Design review of the part built by this model. Coordinates are the model's own, in mm. Face numbers are marked on the shaded views. A direction names the side the tool comes from. Coordinates: 2 decimals unless noted, no trailing zeros. Write each loop counter-clockwise with the first axis right and the second up, starting at its lowest first coordinate (ties: lowest second). Pieces come first, ordered by that corner, then holes. Notation, with made-up numbers: (-5, 56) - (24, 56) arc R18 ccw to (24, 76) - close; hole circle Ø9 at (73.25, 37). An arc over 180 degrees is marked (long way). Use a Markdown table: item, result.
from build123d import *

# Parameters (mm, degrees)
F3_DEPTH = 55.88
F4_COUNT = 15


with BuildPart() as f1:
    # F0 (on Front) → F1 (revolve)
    with BuildSketch(Plane.XZ):
        Polygon((-43.6586365104, 67.430395633), (-43.6586365104, 44.1211201251), (-7.5847627595, 44.1211201251), (-7.5847627595, 11.192150414), (-31.8190082908, 11.192150414), (-31.8190082908, -3.6073876545), (-21.0893414915, -3.6073876545), (-21.0893414915, -7.1222772822), (-15.1695264503, -7.1222772822), (-15.1695264503, -3.6073876545), (-8.6947288364, -3.6073876545), (-8.6947288364, -17.8519431502), (8.1397471949, -17.8519431502), (8.1397471949, -3.6073876545), (16.2794925272, -3.6073876545), (16.2794925272, -7.3072714731), (22.5692950189, -7.3072714731), (22.5692950189, -3.6073876545), (31.8190082908, -3.6073876545), (31.8190082908, 11.192150414), (7.5847627595, 11.192150414), (7.5847627595, 44.1211201251), (43.6586365104, 44.1211201251), (43.6586365104, 67.430395633), align=None)
    revolve(axis=Axis((0, 0, -26.361675933), (1, 0, 0)))

    # F2 (on Right) → F3 (cut, symmetric)
    with BuildSketch(Plane.YZ):
        Polygon((11.4407278597, 52.9837198555), (5.9587107971, 69.429770112), (-5.9587107971, 69.429770112), (-11.4407278597, 52.9837198555), align=None)
    f3 = extrude(amount=F3_DEPTH, both=True, mode=Mode.SUBTRACT)

    # F4: F3 ×15 about axis
    f4_axis = Axis((31.8190082908, 0, -26.361675933), (1, 0, 0))
    for i in range(1, F4_COUNT):
        add(f3.rotate(f4_axis, i * 360 / F4_COUNT), mode=Mode.SUBTRACT)


solid = f1.part
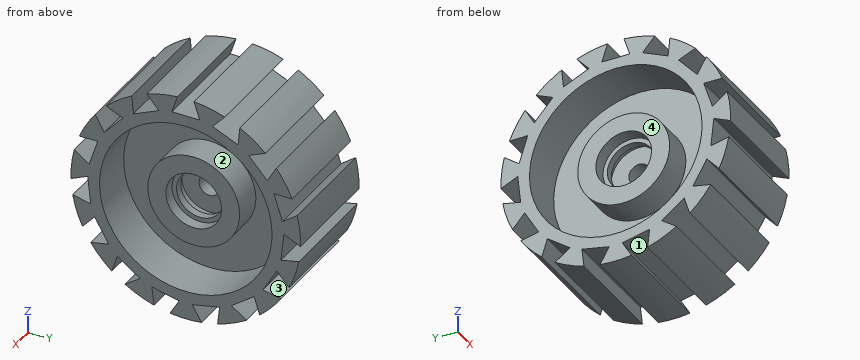
(1) For pin 1 (12 mm diameter, centred on x = 11.5, y = -35.5, fed in from +Z); pin 2 (12 mm diameter, centred on y = -41, z = -0.5, fed in from -X); pin 3 (6 mm diameter, centred on x = -1.5, y = -58.5, fed in from +Z), all flat-tipped, find the tip position at first contact; note any pin that passes through.
Determined:
| item | result |
|---|---|
| pin 1 | z = 62.67 |
| pin 2 | x = -7.58 |
| pin 3 | z = 49.25 |
(2) Take a section at C-C on z = -53.5. Write out the cut boundary in (x, y).
Determined:
| item | result |
|---|---|
| outline | (-43.66, -89.78) - (43.66, -89.78) - (43.66, -65.05) - (7.58, -65.05) - (7.58, -25.96) - (31.82, -25.96) - (31.82, 25.96) - (7.58, 25.96) - (7.58, 65.05) - (43.66, 65.05) - (43.66, 89.78) - (-43.66, 89.78) - (-43.66, 65.05) - (-7.58, 65.05) - (-7.58, 25.96) - (-31.82, 25.96) - (-31.82, -25.96) - (-7.58, -25.96) - (-7.58, -65.05) - (-43.66, -65.05) - close |
(3) For L1, parallel to Z at x = 29.5, y = 0; L2, parallel to Z at x = -19, y = 0; L3, parallel to Z at x = 32.5, y = -40, list the stretches that pass through material, from the lowest coordinate up. Write a range as from..to.
Determined:
| item | result |
|---|---|
| L1 | -120.15..-96.84, -63.92..-49.12, -3.61..11.19, 44.12..52.98 |
| L2 | -120.15..-96.84, -63.92..-45.6, -7.12..11.19, 44.12..52.98 |
| L3 | -111.2..-99.15, -95.38..-84.39, 31.67..42.68 |
(4) Machinability: for the marked faces 1, 2, 3 and 4, which of the approach directions +Z, -Z, +X, -X, +Y, -Y give a long, thin tool a straight path to every point of the face, cutting with its end or side? Answer none if there is none.
Determined:
| item | result |
|---|---|
| face 1 | +X, -X |
| face 2 | +X |
| face 3 | +X, -X, +Y |
| face 4 | -X |
(5) Take a section at B-B on z = 25. Write out the cut boundary in (x, y), and give its area (3 significant figures).
Determined:
| item | result |
|---|---|
| outline | (-43.66, -78.48) - (43.66, -78.48) - (43.66, -70.46) - (-43.66, -70.46) - close; (-43.66, -60.52) - (43.66, -60.52) - (43.66, -48.27) - (7.58, -48.27) - (7.58, 48.27) - (43.66, 48.27) - (43.66, 60.52) - (-43.66, 60.52) - (-43.66, 48.27) - (-7.58, 48.27) - (-7.58, -48.27) - (-43.66, -48.27) - close; (-43.66, 70.46) - (43.66, 70.46) - (43.66, 78.48) - (-43.66, 78.48) - close |
| area | 5,000 mm2 |
(6) Take a section at A-A on x = 29.5. State how many separate pieces and enclosed holes the cut face has, and give its area (3 significant figures).
Determined:
| item | result |
|---|---|
| separate pieces | 2 |
| enclosed holes | 2 |
| area | 10,900 mm2 |
